Part model, mm, in its own coordinate system. Face numbers are marked on the shaded views. A direction names the side the tool comes from. Coordinates: 2 decimals unless noted, no trailing zeros. Loops run counter-clockwise (first coordinate to the right, second up) from the corner with the lowest first, then second, coordinate; pieces in that order, holes last.
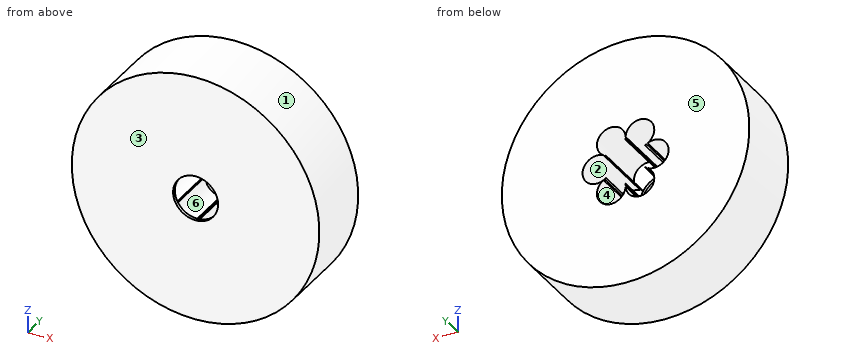
```python
from build123d import *

# Parameters (mm, degrees)
SKETCH1_R           = 27.5
BOSS_EXTRUDE1_DEPTH = 16
SKETCH2_R           = 5
CUT_EXTRUDE1_DEPTH  = 43.053537307
SKETCH3_R           = 3.188575247
CUT_EXTRUDE2_DEPTH  = 15.275638
CIRPATTERN1_START   = 0.7243621
CIRPATTERN1_DEPTH   = 15.2756379


# Read off the part's stored shape, not the designer's step: CirPattern1
with BuildPart() as part:
    # Sketch1 → Boss-Extrude1 (new body)
    with BuildSketch(Plane(origin=(0, 0, 0), x_dir=(1, 0, 0), z_dir=(0, 1, 0))):
        with Locations(Location((0, 0, 0), (0, 0, 270))):
            Circle(SKETCH1_R)
    extrude(amount=BOSS_EXTRUDE1_DEPTH)

    # Sketch2 → Cut-Extrude1 (cut, through all)
    with BuildSketch(Plane(origin=(0, 0, 0), x_dir=(1, 0, 0), z_dir=(0, 1, 0))):
        with Locations(Location((0, 0, 0), (0, 0, 270))):
            Circle(SKETCH2_R)
    extrude(amount=CUT_EXTRUDE1_DEPTH, mode=Mode.SUBTRACT)

    # Sketch3 → Cut-Extrude2 (cut)
    with BuildSketch(Plane(origin=(0, 16, 0), x_dir=(1, 0, 0), z_dir=(0, 1, 0))):
        with Locations((-6.370430977, 0)):
            Circle(SKETCH3_R)
    extrude(amount=-CUT_EXTRUDE2_DEPTH, mode=Mode.SUBTRACT)

    # CirPattern1 outline → CirPattern1 (cut)
    with BuildSketch(Plane(origin=(0, 0, 0), x_dir=(1, 0, 0), z_dir=(0, 1, 0)).offset(CIRPATTERN1_START)):
        with BuildLine():
            ThreePointArc((4.310571121, -2.533569934), (2.5, -4.330127019), (0.038850364, -4.999849063))
            ThreePointArc((0.038850364, -4.999849063), (0.01400188, -5.184665493), (0, -5.370618464))
            ThreePointArc((0, -5.370618464), (-0.01400188, -5.184665493), (-0.038850364, -4.999849063))
            ThreePointArc((-0.038850364, -4.999849063), (-2.5, -4.330127019), (-4.310571121, -2.533569934))
            ThreePointArc((-4.310571121, -2.533569934), (-4.483051087, -2.60445873), (-4.651092024, -2.685309232))
            ThreePointArc((-4.651092024, -2.685309232), (-4.776143353, -2.761387166), (-4.904554442, -2.831645827))
            ThreePointArc((-4.904554442, -2.831645827), (-4.779503112, -8.278342225), (0, -5.663291654))
            ThreePointArc((0, -5.663291654), (4.779503112, -8.278342225), (4.904554442, -2.831645827))
            ThreePointArc((4.904554442, -2.831645827), (9.559006224, 0), (4.904554442, 2.831645827))
            ThreePointArc((4.904554442, 2.831645827), (4.779503112, 8.278342225), (0, 5.663291654))
            ThreePointArc((0, 5.663291654), (-4.779503112, 8.278342225), (-4.904554442, 2.831645827))
            ThreePointArc((-4.904554442, 2.831645827), (-4.776143353, 2.761387166), (-4.651092024, 2.685309232))
            ThreePointArc((-4.651092024, 2.685309232), (-4.483051087, 2.60445873), (-4.310571121, 2.533569934))
            ThreePointArc((-4.310571121, 2.533569934), (-2.5, 4.330127019), (-0.038850364, 4.999849063))
            ThreePointArc((-0.038850364, 4.999849063), (-0.01400188, 5.184665493), (0, 5.370618464))
            ThreePointArc((0, 5.370618464), (0.01400188, 5.184665493), (0.038850364, 4.999849063))
            ThreePointArc((0.038850364, 4.999849063), (2.5, 4.330127019), (4.310571121, 2.533569934))
            ThreePointArc((4.310571121, 2.533569934), (4.483051087, 2.60445873), (4.651092024, 2.685309232))
            ThreePointArc((4.651092024, 2.685309232), (4.497052967, 2.580206763), (4.349421485, 2.466279129))
            ThreePointArc((4.349421485, 2.466279129), (5, 0), (4.349421485, -2.466279129))
            ThreePointArc((4.349421485, -2.466279129), (4.497052967, -2.580206763), (4.651092024, -2.685309232))
            ThreePointArc((4.651092024, -2.685309232), (4.483051087, -2.60445873), (4.310571121, -2.533569934))
        make_face()
    extrude(amount=CIRPATTERN1_DEPTH, mode=Mode.SUBTRACT)


solid = part.part
```
Q1. Mould opens along Z. For the marked faces 1, 2, 3 and 4 say: released by +Z, released by -Z, zero draft, split by the parting line, or undercut.
Q2. Saw through at D-D (x = 11). List the corners of the cut face in (y, z).
Q3. Probe line 1 (X direction, y = 10, z = 0); line 2 (X direction, y = 12.75, z = 8); line 3 (Z direction, x = 6, y = 14). List the from-to ranges inside material, lowest first.
Q4. Saw through at A-A (z = 0). List the corners of the cut face in (x, y).
Q5. Saw through at C-C (z = -11.5). List the corners of the cut face in (x, y).
Q6. Drop flat-ended pins along their axis: P1, Ø5, axis at x = -0.5, z = 1.5, coming from the +Y side; P2, Ø2.5, axis at x = -6.5, z = -0.5, coming from the +Y side; P3, Ø3, axis at x = 8.5, y = 7.5, coming from the +Z side; P4, Ø3, axis at y = 4, z = -22, coming from the -X side. Give the stop position or say it passes through.
Q7. Saw through at B-B (y = 1.75). List the corners of the cut face in (x, z).
Q8. Tool access for the marked faces 5 and 6: list every direction of +Z, -Z, +X, -X, +Y, -Y with a clear straight run to the whole face (end or side of a thin tool).
Checked values:
1. face 1: split by the parting line
1. face 2: undercut
1. face 3: zero draft
1. face 4: undercut
2. outline: (0, -25.2) - (16, -25.2) - (16, 25.2) - (0, 25.2) - close
3. line 1: x = -27.5 to -9.56, 9.56 to 27.5
3. line 2: x = -26.31 to -5.19, -1.18 to 1.18, 5.19 to 26.31
3. line 3: z = -26.84 to -7.01, -4.02 to -3.17, 3.17 to 4.02, 7.01 to 26.84
4. outline: (-27.5, 0) - (-5, 0) - (-5, 0.72) - (-9.56, 0.72) - (-9.56, 16) - (-27.5, 16) - close; (5, 0) - (27.5, 0) - (27.5, 16) - (9.56, 16) - (9.56, 0.72) - (5, 0.72) - close
5. outline: (-24.98, 0) - (24.98, 0) - (24.98, 16) - (-24.98, 16) - close
6. P1: passes through
6. P2: stops at y = 0.72
6. P3: stops at z = 26.59
6. P4: stops at x = -18.33
7. outline: circle Ø55 at (0, 0); (-4.65, -2.69) arc R3.19 cw to (-4.31, -2.53) arc R5 cw to (-4.35, -2.47) arc R3.19 cw to start; (-4.65, 2.69) arc R3.19 cw to (-4.35, 2.47) arc R5 cw to (-4.31, 2.53) arc R3.19 cw to start; (-0.04, -5) arc R3.19 cw to (0, -5.37) arc R3.19 cw to (0.04, -5) arc R5 cw to start; (-0.04, 5) arc R5 cw to (0.04, 5) arc R3.19 cw to (0, 5.37) arc R3.19 cw to start; (4.31, -2.53) arc R3.19 cw to (4.65, -2.69) arc R3.19 cw to (4.35, -2.47) arc R5 cw to start; (4.31, 2.53) arc R5 cw to (4.35, 2.47) arc R3.19 cw to (4.65, 2.69) arc R3.19 cw to start; hole (-4.9, -2.83) arc R3.19 ccw (long way) to (0, -5.66) arc R3.19 ccw (long way) to (4.9, -2.83) arc R3.19 ccw (long way) to (4.9, 2.83) arc R3.19 ccw (long way) to (0, 5.66) arc R3.19 ccw (long way) to (-4.9, 2.83) arc R3.19 ccw (long way) to start
8. face 5: +Z, -Z, +X, -X, +Y
8. face 6: +Y
